from build123d import *
from OCP.BRepFilletAPI import BRepFilletAPI_MakeChamfer

# Parameters (mm, degrees)
SKETCH1_W           = 215.9
SKETCH1_H           = 228.6
BOSS_EXTRUDE1_DEPTH = 3.175
SKETCH2_R           = 17.145
CUT_EXTRUDE1_DEPTH  = 315.453256661
SKETCH3_R           = 1.5875
CUT_EXTRUDE2_DEPTH  = 315.453256661
SKETCH4_R           = 1.5875
CUT_EXTRUDE3_DEPTH  = 315.453256661
CHAMFER1_SIZE       = 2.1082
CHAMFER1_SIZE2      = 1.832630301
SKETCH5_W           = 25.4
SKETCH5_H           = 50.8
SKETCH5_H_2         = 25.4
SKETCH5_W_2         = 50.8
SKETCH5_W_3         = 76.2
SKETCH5_H_3         = 88.9
CUT_EXTRUDE4_DEPTH  = 1.5875
FILLET1_R           = 3.175
FILLET2_R           = 25.4


with BuildPart() as part:
    # Sketch1 → Boss-Extrude1 (new body)
    with BuildSketch(Plane(origin=(0, 0, 0), x_dir=(1, 0, 0), z_dir=(0, 1, 0))):
        with Locations((107.95, 114.3)):
            Rectangle(SKETCH1_W, SKETCH1_H)
    extrude(amount=BOSS_EXTRUDE1_DEPTH)

    # Sketch2 → Cut-Extrude1 (cut, through all)
    with BuildSketch(Plane(origin=(0, 3.175, 0), x_dir=(1, 0, 0), z_dir=(0, 1, 0))):
        with Locations(Location((139.7, 38.1, 0), (0, 0, 270))):
            Circle(SKETCH2_R)
        with Locations(Location((76.2, 38.1, 0), (0, 0, 270))):
            Circle(SKETCH2_R)
    extrude(amount=-CUT_EXTRUDE1_DEPTH, mode=Mode.SUBTRACT)

    # Sketch3 → Cut-Extrude2 (cut, through all)
    with BuildSketch(Plane(origin=(0, 3.175, 0), x_dir=(1, 0, 0), z_dir=(0, 1, 0))):
        with Locations(Location((107.95, 130.81, 0), (0, 0, 270))):
            Circle(SKETCH3_R)
        with Locations(Location((122.248079416, 106.045, 0), (0, 0, 270))):
            Circle(SKETCH3_R)
        with Locations(Location((93.651920584, 106.045, 0), (0, 0, 270))):
            Circle(SKETCH3_R)
    extrude(amount=-CUT_EXTRUDE2_DEPTH, mode=Mode.SUBTRACT)

    # Sketch4 → Cut-Extrude3 (cut, through all)
    with BuildSketch(Plane(origin=(0, 3.175, 0), x_dir=(1, 0, 0), z_dir=(0, 1, 0))):
        with Locations(Location((6.35, 146.05, 0), (0, 0, 270))):
            Circle(SKETCH4_R)
        with Locations(Location((6.35, 82.55, 0), (0, 0, 270))):
            Circle(SKETCH4_R)
        with Locations(Location((57.15, 6.35, 0), (0, 0, 270))):
            Circle(SKETCH4_R)
        with Locations(Location((57.15, 222.25, 0), (0, 0, 270))):
            Circle(SKETCH4_R)
        with Locations(Location((158.75, 6.35, 0), (0, 0, 90))):
            Circle(SKETCH4_R)
        with Locations(Location((209.55, 82.55, 0), (0, 0, 90))):
            Circle(SKETCH4_R)
        with Locations(Location((209.55, 146.05, 0), (0, 0, 90))):
            Circle(SKETCH4_R)
        with Locations(Location((158.75, 222.25, 0), (0, 0, 90))):
            Circle(SKETCH4_R)
    extrude(amount=-CUT_EXTRUDE3_DEPTH, mode=Mode.SUBTRACT)

    # Chamfer1: one chamfer whose edges measure the first distance from different faces: ONE call of the kernel's chamfer builder (chamfer() names one face for all edges)
    chamfer1_edges_1 = [part.edges().sort_by_distance(p)[0] for p in [
        (107.95, 0, -132.3975),
    ]]
    chamfer1_side_1 = [part.faces().sort_by_distance(p)[0] for p in [
        (107.95, 1.5875, -132.3975),
    ]]
    chamfer1_edges_2 = [part.edges().sort_by_distance(p)[0] for p in [
        (122.248079416, 0, -107.6325),
    ]]
    chamfer1_side_2 = [part.faces().sort_by_distance(p)[0] for p in [
        (122.248079416, 1.5875, -107.6325),
    ]]
    chamfer1_edges_3 = [part.edges().sort_by_distance(p)[0] for p in [
        (93.651920584, 0, -107.6325),
    ]]
    chamfer1_side_3 = [part.faces().sort_by_distance(p)[0] for p in [
        (93.651920584, 1.5875, -107.6325),
    ]]
    chamfer1 = BRepFilletAPI_MakeChamfer(part.part.solid().wrapped)
    for e in chamfer1_edges_1:
        chamfer1.Add(CHAMFER1_SIZE, CHAMFER1_SIZE2, e.wrapped, chamfer1_side_1[0].wrapped)  # the first distance lies on this face
    for e in chamfer1_edges_2:
        chamfer1.Add(CHAMFER1_SIZE, CHAMFER1_SIZE2, e.wrapped, chamfer1_side_2[0].wrapped)  # the first distance lies on this face
    for e in chamfer1_edges_3:
        chamfer1.Add(CHAMFER1_SIZE, CHAMFER1_SIZE2, e.wrapped, chamfer1_side_3[0].wrapped)  # the first distance lies on this face
    add(Compound.cast(chamfer1.Shape()), mode=Mode.REPLACE)

    # Sketch5 → Cut-Extrude4 (cut)
    with BuildSketch(Plane.XZ):
        with Locations((31.75, -44.45)):
            Rectangle(SKETCH5_W, SKETCH5_H)
        with Locations((31.75, -82.55)):
            Rectangle(SKETCH5_W, SKETCH5_H_2)
        with Locations((69.85, -82.55)):
            Rectangle(SKETCH5_W_2, SKETCH5_H_2)
        with Locations((57.15, -165.1)):
            Rectangle(SKETCH5_W_3, SKETCH5_H_3)
        with Locations((158.75, -165.1)):
            Rectangle(SKETCH5_W_3, SKETCH5_H_3)
        with Locations((146.05, -82.55)):
            Rectangle(SKETCH5_W_2, SKETCH5_H_2)
        with Locations((184.15, -82.55)):
            Rectangle(SKETCH5_W, SKETCH5_H_2)
        with Locations((184.15, -44.45)):
            Rectangle(SKETCH5_W, SKETCH5_H)
    extrude(amount=-CUT_EXTRUDE4_DEPTH, mode=Mode.SUBTRACT)

    # Fillet1
    fillet1_edges = [part.edges().sort_by_distance(p)[0] for p in [
        (120.65, 0.79375, -120.65),
        (196.85, 0.79375, -120.65),
        (196.85, 0.79375, -209.55),
        (120.65, 0.79375, -209.55),
        (19.05, 0.79375, -120.65),
        (95.25, 0.79375, -120.65),
        (95.25, 0.79375, -209.55),
        (19.05, 0.79375, -209.55),
        (19.05, 0.79375, -95.25),
        (19.05, 0.79375, -19.05),
        (44.45, 0.79375, -19.05),
        (95.25, 0.79375, -69.85),
        (95.25, 0.79375, -95.25),
        (196.85, 0.79375, -95.25),
        (120.65, 0.79375, -95.25),
        (120.65, 0.79375, -69.85),
        (171.45, 0.79375, -19.05),
        (196.85, 0.79375, -19.05),
    ]]
    fillet(fillet1_edges, radius=FILLET1_R)

    # Fillet2
    fillet2_edges = [part.edges().sort_by_distance(p)[0] for p in [
        (44.45, 0.79375, -69.85),
        (171.45, 0.79375, -69.85),
    ]]
    fillet(fillet2_edges, radius=FILLET2_R)


solid = part.part
Model file for the job. Use its own axes, mm. A direction names the side the tool comes from. Give positions to 0.01 mm unless a question says otherwise; leave off trailing zeros.
Item 1: Which spindle directions (+Z, -Z, +X, -X, +Y, -Y) get a long thin tool onto all of the face, cutting with end or side? Do faces 3 (the face through (106, 3.175, -116)), 4 (the face through (158, 1.588, -164)). Say none if no direction does.
Check values:
face 3: +Z, -Z, +X, -X, +Y
face 4: -Y
Item 2: Drill centre lines: line 1 along X through (y, z) = (1.7, -222.25); line 2 along X through (y, z) = (1, -207); line 3 along Z through (x, y) = (180.5, 0.8). Where is each one in solid material? Low to high.
Check values:
line 1: x = 0 to 55.56, 58.74 to 157.16, 160.34 to 215.9
line 2: x = 0 to 19.11, 95.19 to 120.71, 196.79 to 215.9
line 3: z = -228.6 to -209.55, -120.65 to -95.25, -19.05 to 0
Item 3: Drop flat-ended pins along their axis: P1, Ø1.3, axis at y = 1, z = -84.5, coming from the -X side; P2, Ø3.5, axis at x = 93.65, z = -106.04, coming from the -Y side; P3, Ø1, axis at x = 160.5, z = -180, coming from the -Y side; P4, Ø5, axis at x = 107.95, z = -130.81, coming from the -Y side. Give the stop position or say it passes through.
Check values:
P1: stops at x = 0
P2: stops at y = 1.92
P3: stops at y = 1.59
P4: stops at y = 1.06
Item 4: Slice it at A-A (z = -38.1). Give the number of separate pieces and of enclosed holes in the cut face, plus the area to 3 significant figures.
Check values:
separate pieces: 3
enclosed holes: 0
area: 387 mm2
Item 5: Mould opens along X. For faces 1 (the face through (57, 1.588, -164)), 2 (the face through (106, 0, -116)) say: +X half, -X half, draft (parallel to the pull), parting line (faces both ways), or undercut.
Check values:
face 1: undercut
face 2: draft
